```python
from build123d import *

# Parameters (mm, degrees)
BOSS_EXTRUDE1_DEPTH = 24.1
SKETCH2_W           = 20.1
SKETCH2_H           = 6.5
CUT_EXTRUDE1_DEPTH  = 9.65
SKETCH3_W           = 1.5
SKETCH3_H           = 3
CUT_EXTRUDE2_DEPTH  = 28.965916756
SKETCH4_R           = 3
CUT_EXTRUDE3_DEPTH  = 2.8
CUT_EXTRUDE4_DEPTH  = 30.291124936
CHAMFER1_SIZE       = 1


with BuildPart() as part:
    # Sketch1 → Boss-Extrude1 (new body)
    with BuildSketch(Plane.XY):
        Polygon((0, 8.5), (1.5, 8.5), (3.4, 10.4), (5.4, 10.4), (7.3, 8.5), (13, 8.5), (13, 0), (7.3, 0), (5.4, -1.9), (3.4, -1.9), (1.5, 0), (0, 0), align=None)
    extrude(amount=BOSS_EXTRUDE1_DEPTH)

    # Sketch2 → Cut-Extrude1 (cut)
    with BuildSketch(Plane(origin=(13, 0, 0), x_dir=(0, 0, -1), z_dir=(1, 0, 0))):
        with Locations((-12.05, 4.25)):
            Rectangle(SKETCH2_W, SKETCH2_H)
    extrude(amount=-CUT_EXTRUDE1_DEPTH, mode=Mode.SUBTRACT)

    # Sketch3 → Cut-Extrude2 (cut, through all)
    with BuildSketch(Plane(origin=(3.35, 0, 0), x_dir=(0, 0, -1), z_dir=(1, 0, 0))):
        with Locations((-4.75, 4.25)):
            Rectangle(SKETCH3_W, SKETCH3_H)
        with Locations((-19.75, 4.25)):
            Rectangle(SKETCH3_W, SKETCH3_H)
        with Locations((-12.25, 4.25)):
            Rectangle(SKETCH3_W, SKETCH3_H)
    extrude(amount=-CUT_EXTRUDE2_DEPTH, mode=Mode.SUBTRACT)

    # Sketch4 → Cut-Extrude3 (cut)
    with BuildSketch(Plane.ZY):
        with Locations((8, 4.25)):
            Circle(SKETCH4_R)
        with Locations((16.5, 4.25)):
            Circle(SKETCH4_R)
    extrude(amount=-CUT_EXTRUDE3_DEPTH, mode=Mode.SUBTRACT)

    # Sketch5 → Cut-Extrude4 (cut, through all)
    with BuildSketch(Plane.ZY):
        Polygon((24.1, -1.9), (24.1, 0.6), (21.6, -1.9), align=None)
        Polygon((21.6, 10.4), (24.1, 10.4), (24.1, 7.9), align=None)
    extrude(amount=-CUT_EXTRUDE4_DEPTH, mode=Mode.SUBTRACT)

    # Chamfer1
    chamfer1_edges = [part.edges().sort_by_distance(p)[0] for p in [
        (0, 8.5, 11.75),
        (0, 0, 11.75),
    ]]
    chamfer(chamfer1_edges, length=CHAMFER1_SIZE)


solid = part.part
```
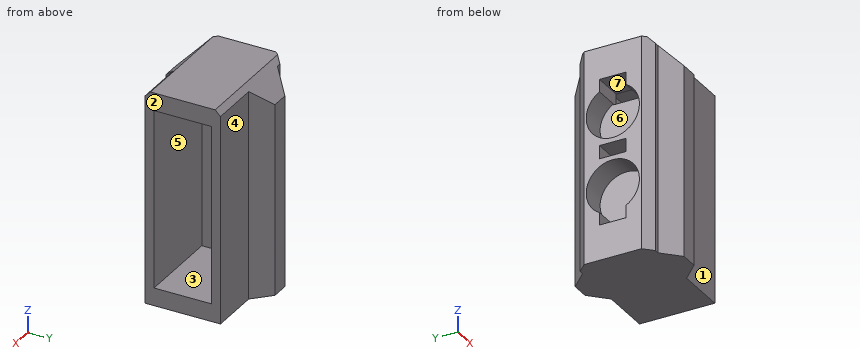
Model file for the job. Use its own axes, mm. Face numbers are marked on the shaded views. A direction names the side the tool comes from. Give positions to 0.01 mm unless a question says otherwise; leave off trailing zeros. Write each loop counter-clockwise with the first axis right and the second up, starting at its lowest first coordinate (ties: lowest second). Pieces come first, ordered by that corner, then holes. Notation, with made-up numbers: (-16.75, 38) -> (18.25, 38) arc R27 ccw to (18.25, 56) -> close; hole circle Ø2 at (0, 85.25). An arc over 180 degrees is marked (long way). Use CSV: the item, a comma, the result in double quotes. Start each with the question number.
1) Drill centre lines: L1, parallel to Z at x = 1.65, y = 4.25; L2, parallel to Y at x = 11, z = 13; L3, parallel to Z at x = 3.75, y = 2.25. Where is each one in solid material? Low to high.
2) Cut at A-A on y = 4.25. List the corners of the cut face in (x, z).
3) Tool access for the marked faces 5, 6 and 7: list every direction of +Z, -Z, +X, -X, +Y, -Y with a clear straight run to the whole face (end or side of a thin tool).
4) Two-plate mould, pull along Y, no slides. Class the marked faces 1, 2, 3 and 4: released by +Y, released by -Y, zero draft, split by the parting line, or undercut.
5) Pin check, flat tips, straight feed: P1, Ø3, axis at x = 11, z = 12, coming from the -Y side; P2, Ø1.2, axis at x = 2, z = 5, coming from the +Y side; P3, Ø1.2, axis at x = 1.5, z = 12.5, coming from the +Y side. Stop position of each tip, or through.
6) Cut at C-C on z = 16.5. List the corners of the cut face in (x, y).
7) Cut at D-D on x = 4.25. List the corners of the cut face in (y, z), plus the area to 3 significant figures.
8) Cut at B-B on x = 7. List the corners of the cut face in (y, z).
Final values:
1,L1,"z = 0 to 4, 11 to 11.5, 13 to 13.5, 20.5 to 24.1"
1,L2,"y = 0 to 1, 7.5 to 8.5"
1,L3,"z = 0 to 2, 22.1 to 24.1"
2,outline,"(0, 0) -> (13, 0) -> (13, 2) -> (3.35, 2) -> (3.35, 4) -> (0, 4) -> close; (0, 11) -> (2.8, 11) -> (2.8, 5.5) -> (3.35, 5.5) -> (3.35, 11.5) -> (0, 11.5) -> close; (0, 13) -> (3.35, 13) -> (3.35, 19) -> (2.8, 19) -> (2.8, 13.5) -> (0, 13.5) -> close; (0, 20.5) -> (3.35, 20.5) -> (3.35, 22.1) -> (13, 22.1) -> (13, 24.1) -> (0, 24.1) -> close"
3,face 5,"+X"
3,face 6,"-X"
3,face 7,"+X, -X"
4,face 1,"released by -Y"
4,face 2,"zero draft"
4,face 3,"undercut"
4,face 4,"released by +Y"
5,P1,"stops at y = 0"
5,P2,"stops at y = 9.6"
5,P3,"stops at y = 9.1"
6,outline,"(0, 1) -> (1, 0) -> (1.5, 0) -> (3.4, -1.9) -> (5.4, -1.9) -> (7.3, 0) -> (13, 0) -> (13, 1) -> (3.35, 1) -> (3.35, 7.5) -> (13, 7.5) -> (13, 8.5) -> (7.3, 8.5) -> (5.4, 10.4) -> (3.4, 10.4) -> (1.5, 8.5) -> (1, 8.5) -> (0, 7.5) -> (0, 7.25) -> (2.8, 7.25) -> (2.8, 1.25) -> (0, 1.25) -> close"
7,outline,"(-1.9, 0) -> (10.4, 0) -> (10.4, 21.6) -> (7.9, 24.1) -> (0.6, 24.1) -> (-1.9, 21.6) -> close; hole (1, 2) -> (7.5, 2) -> (7.5, 22.1) -> (1, 22.1) -> close"
7,area,"160 mm2"
8,outline,"(-0.3, 0) -> (8.8, 0) -> (8.8, 23.2) -> (7.9, 24.1) -> (0.6, 24.1) -> (-0.3, 23.2) -> close; hole (1, 2) -> (7.5, 2) -> (7.5, 22.1) -> (1, 22.1) -> close"
